Geometry: final body of the model. Coordinates: model frame, mm. Face numbers are marked on the shaded views. A direction names the side the tool comes from. Coordinates: 2 decimals unless noted, no trailing zeros. Write each loop counter-clockwise with the first axis right and the second up, starting at its lowest first coordinate (ties: lowest second). Pieces come first, ordered by that corner, then holes. Notation, with made-up numbers: (-16.5, 89.25) -> (-6.5, 89.25) arc R25 ccw to (-6.5, 122.25) -> close; hole circle Ø10 at (27.5, 18.5). An arc over 180 degrees is marked (long way). Answer as a JSON object with one key per item and string values. Group by question number.
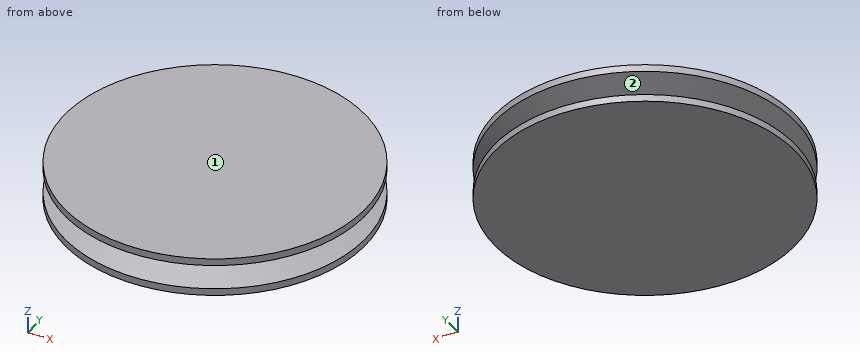
Autodesk Inventor part; units mm, degrees
ref_plane "Plano de correa" through (0, 64, 10) normal (0, 0, 1) x (1, 0, 0)
ref_plane "YZ Plane" through (0, 0, 0) normal (1, 0, 0) x (0, 1, 0)
ref_plane "XZ Plane" through (0, 0, 0) normal (0, 1, 0) x (-1, 0, 0)
sketch "Boceto principal" plane through (0, 0, 0) normal (1, 0, 0) x (0, 1, 0)
  line L0 (0, 20) -> (77.8, 20)
  line L1 (77.8, 20) -> (77.8, 16.356)
  line L2 (77.8, 16.356) -> (64, 12.137)
  line L3 (64, 12.137) -> (64, 7.863)
  line L4 (64, 7.863) -> (77.8, 3.644)
  line L5 (77.8, 3.644) -> (77.8, 0)
  line L6 (77.8, 0) -> (0, 0)
  line L7 (75, 15.5) -> (75, 4.5) construction
  line L8 (64, 10) -> (75, 10) construction
  line L9 (77.8, 16.356) -> (77.8, 3.644)
  line L10 (0, -4) -> (0, 24)
  line L11 (0, 0) -> (0, 20)
  dimension "d0" = 11
  dimension "d1" = 34
  dimension "d2" = 2.8
  dimension "d6" = 20
  dimension "d21" = 150
  dimension "d25" = 13.8
  dimension "d27" = 10
ref_plane "Plano de correa" through (0, 64, 10) normal (0, 0, 1) x (1, 0, 0)
revolve "Cuerpo" add sketch "Boceto principal" angle 360 about axis through (0, 0, -10) along (0, 0, 1)
revolve "Para ranuras" cut sketch "Boceto principal" angle 360 about axis through (0, 0, -10) along (0, 0, 1) contours L9 L4 L3 L2
fillet "Empalme externo" [suppressed]
fillet "Empalme interno" [suppressed]
pattern_of_one "Patrón para ranuras"
equation "\"d0\" = da_Bw"
equation "\"d1\" = da_Alfa"
equation "\"d2\" = da_c"
equation "\"d21\" = da_Dw"
equation "\"d25\" = da_Hd"
equation "\"d27\" = da_Se"
equation "\"da_r1\" = 0"
equation "\"da_r2\" = 0"
equation "\"d18\" = da_Sg"
equation "\"da_Bw\" = 11"
equation "\"da_Alfa\" = 34deg"
equation "\"da_c\" = 2.8"
equation "\"da_Dw\" = 150"
equation "\"da_Hd\" = 13.8"
equation "\"da_Se\" = 10"
equation "\"da_Sg\" = 15"
properties part number "Polea ranurada1" material "Steel"
Item 1: Contact query for flat-ended pins moving along their axis: pin 1 (1.5 mm diameter, centred on y = -40.5, z = 16.5, fed in from -X); pin 2 (10 mm diameter, centred on x = -28.5, y = 32.5, fed in from -Z); pin 3 (12 mm diameter, centred on x = -19.5, z = 10.5, fed in from +Y). Output: stop coordinate, or through.
Item 2: Section A-A on x = 0. Output: boundary loops of the cut face in (y, z), then the cut area to 3 significant figures.
Item 3: Section C-C on z = 14.25. Output: boundary loops of the cut face in (x, y), then the cut area to 3 significant figures.
Item 4: Ray query, L1, parallel to Z at x = 47.5, y = -59.5; L2, parallel to Z at x = 67.5, y = 17; L3, parallel to Y at x = -12, z = 18. Return the intervals inside material, ascending. Write a range as [from, to].
Item 5: Set-up query: the marked faces 1 and 2. Return all of +Z, -Z, +X, -X, +Y, -Y with unobstructed straight access to the full face (end or side cutting, diameter ignored); none if empty.
Answer sheet:
{
 "1": {"pin 1": "stops at x = -66.88", "pin 2": "stops at z = 0", "pin 3": "stops at y = 75.64"},
 "2": {"outline": "(-77.8, 0) -> (77.8, 0) -> (77.8, 3.64) -> (64, 7.86) -> (64, 12.14) -> (77.8, 16.36) -> (77.8, 20) -> (-77.8, 20) -> (-77.8, 16.36) -> (-64, 12.14) -> (-64, 7.86) -> (-77.8, 3.64) -> close", "area": "2,880 mm^2"},
 "3": {"outline": "circle Ø141.82 at (0, 0)", "area": "15,800 mm^2"},
 "4": {"L1": "z = [0, 4.15], [15.85, 20]", "L2": "z = [0, 6.15], [13.85, 20]", "L3": "y = [-76.87, 76.87]"},
 "5": {"face 1": "+Z, +X, -X, +Y, -Y", "face 2": "none"}
}
